Work out the finished part from the listing and answer in its coordinate system (mm). Face numbers are marked on the shaded views. A direction names the side the tool comes from. Coordinates: 2 decimals unless noted, no trailing zeros. Loops run counter-clockwise (first coordinate to the right, second up) from the corner with the lowest first, then second, coordinate; pieces in that order, holes last. Notation, with made-up numbers: (-2.75, -23) - (18.25, -23) arc R26 ccw to (18.25, 4) - close; hole circle Ø5 at (63.25, 5). An arc over 180 degrees is marked (long way). Write each question's results on one line, items separated by ' | '. Start each with the question number.
1. Which of the six approach directions +Z, -Z, +X, -X, +Y, -Y give full straight-line access (tool end or side, diameter ignored) to the marked faces 1, 2 and 3?
2. A cutting plane is placed at B-B on z = 1. State how many separate pieces and enclosed holes the cut face has, then the cut area to 3 significant figures.
3. Find the intervals of material crossed by line 1 along X through (y, z) = (-13.5, 0.3); line 2 along X through (y, z) = (0.5, 1.95); line 3 along X through (y, z) = (-34.5, 1.05), in increasing order. Write a range as [from, to].
4. This flat-tipped pin is pushed along its axis until it touches: P1, Ø12.5, axis at x = 18.5, y = -7, coming from the -Z side. Where does it stop, or does it pass through?
5. Determine the mould class of the marked faces 4 and 5 for opening direction Y: released by +Y, released by -Y, zero draft, split by the parting line, or undercut.
6. A cutting plane is placed at A-A on x = 41. Determine the outline of the cut face in (y, z) (3 decimals), then the cut area to 3 significant figures.
from build123d import *

# Parameters (mm, degrees)
BOSS_EXTRUDE1_DEPTH = 3
SKETCH2_R           = 1.5
CUT_EXTRUDE1_DEPTH  = 10
SKETCH6_W           = 23
SKETCH6_H           = 1.5
CUT_EXTRUDE2_DEPTH  = 20
SKETCH7_W           = 66.1
SKETCH7_H           = 41.35
CUT_EXTRUDE3_DEPTH  = 1.5
SKETCH9_R           = 0.85
CUT_EXTRUDE4_DEPTH  = 6.5
SKETCH10_W          = 43
SKETCH10_H          = 43
CUT_EXTRUDE5_DEPTH  = 1.5
SKETCH17_R          = 1.5
CUT_EXTRUDE11_DEPTH = 30.5
SKETCH18_R          = 1.5
CUT_EXTRUDE12_DEPTH = 30.5
SKETCH19_W          = 28
SKETCH19_H          = 41.645525892
CUT_EXTRUDE13_DEPTH = 1.5
SKETCH20_R          = 1.5
CUT_EXTRUDE14_DEPTH = 1.5
SKETCH21_R          = 1.5
CUT_EXTRUDE15_DEPTH = 10
SKETCH23_R          = 5.75
CUT_EXTRUDE16_DEPTH = 4


with BuildPart() as part:
    # Sketch1 → Boss-Extrude1 (new body)
    with BuildSketch(Plane.XY):
        with BuildLine():
            Line((-65.435778714, 44.275111174), (0, 50))
            Line((0, 50), (95, 50))
            ThreePointArc((95, 50), (98.535533906, 48.535533906), (100, 45))
            Line((100, 45), (100, -45))
            ThreePointArc((100, -45), (98.535533906, -48.535533906), (95, -50))
            Line((95, -50), (0, -50))
            Line((0, -50), (-65.435778714, -44.275111174))
            ThreePointArc((-65.435778714, -44.275111174), (-68.686386684, -42.672088721), (-70, -39.294137683))
            Line((-70, -39.294137683), (-70, 39.294137683))
            ThreePointArc((-70, 39.294137683), (-68.686386684, 42.672088721), (-65.435778714, 44.275111174))
        make_face()
    extrude(amount=BOSS_EXTRUDE1_DEPTH)

    # Sketch2 → Cut-Extrude1 (cut)
    with BuildSketch(Plane.XY.offset(3)):
        with Locations((-48, -40)):
            Circle(SKETCH2_R)
        with Locations((-29, -40)):
            Circle(SKETCH2_R)
        with Locations((-48, 40)):
            Circle(SKETCH2_R)
        with Locations((-29, 40)):
            Circle(SKETCH2_R)
    extrude(amount=-CUT_EXTRUDE1_DEPTH, mode=Mode.SUBTRACT)

    # Sketch6 → Cut-Extrude2 (cut)
    with BuildSketch(Plane(origin=(0, 50, 0), x_dir=(1, 0, 0), z_dir=(0, 1, 0))):
        with Locations((-38.5, -0.75)):
            Rectangle(SKETCH6_W, SKETCH6_H)
    cut_extrude2 = extrude(amount=-CUT_EXTRUDE2_DEPTH, mode=Mode.SUBTRACT)

    # Sketch7 → Cut-Extrude3 (cut)
    with BuildSketch(Plane(origin=(0, 0, 0), x_dir=(-1, 0, 0), z_dir=(0, 0, -1))):
        with Locations((-27.95, 0)):
            Rectangle(SKETCH7_W, SKETCH7_H)
    extrude(amount=-CUT_EXTRUDE3_DEPTH, mode=Mode.SUBTRACT)

    # Sketch9 → Cut-Extrude4 (cut)
    with BuildSketch(Plane(origin=(0, 0, 0), x_dir=(-1, 0, 0), z_dir=(0, 0, -1))):
        with Locations((-54.5, 9.925)):
            Circle(SKETCH9_R)
        with Locations((-54.5, -5.375)):
            Circle(SKETCH9_R)
        with Locations((-13.8, 9.925)):
            Circle(SKETCH9_R)
        with Locations((-13.8, -5.375)):
            Circle(SKETCH9_R)
    extrude(amount=-CUT_EXTRUDE4_DEPTH, mode=Mode.SUBTRACT)

    # Sketch10 → Cut-Extrude5 (cut)
    with BuildSketch(Plane(origin=(0, 0, 0), x_dir=(-1, 0, 0), z_dir=(0, 0, -1))):
        with Locations((28.6, 0)):
            Rectangle(SKETCH10_W, SKETCH10_H)
    extrude(amount=-CUT_EXTRUDE5_DEPTH, mode=Mode.SUBTRACT)

    # Mirror1: Cut-Extrude2 across plane
    add(cut_extrude2.mirror(Plane.ZX), mode=Mode.SUBTRACT)

    # Sketch17 → Cut-Extrude11 (cut)
    with BuildSketch(Plane(origin=(0, 0, 0), x_dir=(-1, 0, 0), z_dir=(0, 0, -1))):
        with Locations((-36.309541126, -36.85)):
            Circle(SKETCH17_R)
        with Locations((-36.309541126, 36.85)):
            Circle(SKETCH17_R)
    extrude(amount=-CUT_EXTRUDE11_DEPTH, mode=Mode.SUBTRACT)

    # Sketch18 → Cut-Extrude12 (cut)
    with BuildSketch(Plane(origin=(0, 0, 0), x_dir=(-1, 0, 0), z_dir=(0, 0, -1))):
        with Locations((-95, -36.5)):
            Circle(SKETCH18_R)
        with Locations((-95, 36.5)):
            Circle(SKETCH18_R)
        with Locations((60, -23.5)):
            Circle(SKETCH18_R)
        with Locations((60, 23.5)):
            Circle(SKETCH18_R)
    extrude(amount=-CUT_EXTRUDE12_DEPTH, mode=Mode.SUBTRACT)

    # Sketch19 → Cut-Extrude13 (cut)
    with BuildSketch(Plane(origin=(0, 0, 0), x_dir=(-1, 0, 0), z_dir=(0, 0, -1))):
        with Locations((-76, 0)):
            Rectangle(SKETCH19_W, SKETCH19_H)
    extrude(amount=-CUT_EXTRUDE13_DEPTH, mode=Mode.SUBTRACT)

    # Sketch20 → Cut-Extrude14 (cut)
    with BuildSketch(Plane(origin=(0, 0, 1.5), x_dir=(-1, 0, 0), z_dir=(0, 0, -1))):
        with Locations((-66, 0)):
            Circle(SKETCH20_R)
        with Locations((-85.28, 0)):
            Circle(SKETCH20_R)
    extrude(amount=-CUT_EXTRUDE14_DEPTH, mode=Mode.SUBTRACT)

    # Sketch21 → Cut-Extrude15 (cut)
    with BuildSketch(Plane.XY.offset(3)):
        with Locations((-42.8, 30.1)):
            Circle(SKETCH21_R)
        with Locations((-42.8, -29.5)):
            Circle(SKETCH21_R)
    extrude(amount=-CUT_EXTRUDE15_DEPTH, mode=Mode.SUBTRACT)

    # Sketch23 → Cut-Extrude16 (cut)
    with BuildSketch(Plane(origin=(0, 50, 0), x_dir=(1, 0, 0), z_dir=(0, 1, 0))):
        with Locations((75.64, 3)):
            Circle(SKETCH23_R)
    cut_extrude16 = extrude(amount=-CUT_EXTRUDE16_DEPTH, mode=Mode.SUBTRACT)

    # Mirror2: Cut-Extrude16 across plane
    add(cut_extrude16.mirror(Plane.ZX), mode=Mode.SUBTRACT)


solid = part.part
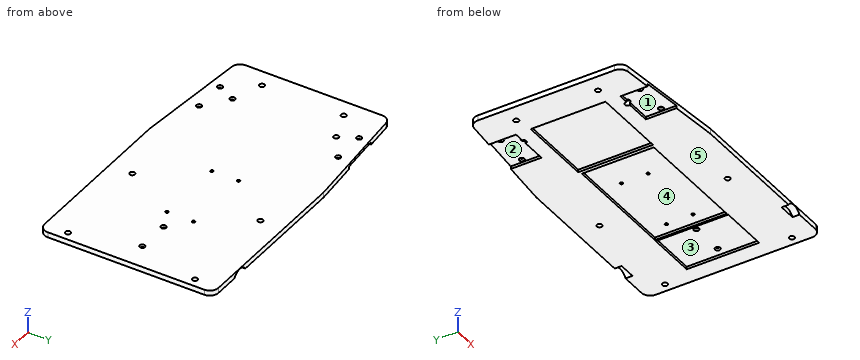
Values:
1) face 1: -Z, -Y | face 2: -Z, +Y | face 3: -Z
2) separate pieces: 1 | enclosed holes: 9 | area: 9,920 mm^2
3) line 1: [-70, -50.1], [-7.1, -5.1], [61, 62], [90, 100] | line 2: [-70, 64.59], [67.41, 83.87], [86.69, 100] | line 3: [-70, -50], [-27, 100]
4) P1: z = 1.5
5) face 4: undercut | face 5: zero draft
6) outline: (-50, 0) - (-20.675, 0) - (-20.675, 1.5) - (20.675, 1.5) - (20.675, 0) - (50, 0) - (50, 3) - (-50, 3) - close | area: 238 mm^2
